```python
from build123d import *

# Parameters (mm, degrees)
MAIN_BODY_DEPTH          = 30.5
SKETCH2_R                = 4.23
LONG_SHAFT_COLLAR_DEPTH  = 2
SKETCH3_R                = 1
LONG_SHAFT_DEPTH         = 10.3
SKETCH5_W                = 8.3
SKETCH5_H                = 5.6
LEAD_BUMP_DEPTH          = 1.15
SKETCH6_R                = 3.075
SHORT_SHAFT_COLLAR_DEPTH = 1.5
SHORT_START              = 5.5
SKETCH7_R                = 1
SHORT_SHAFT_DEPTH        = 5.5


with BuildPart() as part:
    # Sketch1 → Main Body (new body)
    with BuildSketch(Plane.XY):
        with BuildLine():
            Line((-7.867656894, -9.16), (7.867656894, -9.16))
            ThreePointArc((7.867656894, -9.16), (12.075, 0), (7.867656894, 9.16))
            Line((7.867656894, 9.16), (-7.867656894, 9.16))
            ThreePointArc((-7.867656894, 9.16), (-12.075, 0), (-7.867656894, -9.16))
        make_face()
    extrude(amount=MAIN_BODY_DEPTH)

    # Sketch2 → Long Shaft Collar (add)
    with BuildSketch(Plane(origin=(0, 0, 0), x_dir=(-1, 0, 0), z_dir=(0, 0, -1))):
        Circle(SKETCH2_R)
    extrude(amount=LONG_SHAFT_COLLAR_DEPTH)

    # Sketch3 → Long Shaft (add)
    with BuildSketch(Plane(origin=(0, 0, -2), x_dir=(-1, 0, 0), z_dir=(0, 0, -1))):
        with Locations(Location((0, 0, 0), (0, 0, 180))):
            Circle(SKETCH3_R)
    extrude(amount=LONG_SHAFT_DEPTH)

    # Sketch5 → Lead Bump (add)
    with BuildSketch(Plane(origin=(0, 9.16, 0), x_dir=(1, 0, 0), z_dir=(0, 1, 0))):
        with Locations((0, -2.8)):
            Rectangle(SKETCH5_W, SKETCH5_H)
    extrude(amount=LEAD_BUMP_DEPTH)

    # Sketch6 → Short Shaft Collar (add)
    with BuildSketch(Plane.XY.offset(30.5)):
        Circle(SKETCH6_R)
    extrude(amount=SHORT_SHAFT_COLLAR_DEPTH)

    # Sketch7 → Short shaft (add)
    with BuildSketch(Plane.XY.offset(32).offset(SHORT_START)):
        Circle(SKETCH7_R)
    extrude(amount=-SHORT_SHAFT_DEPTH)


solid = part.part
```
Geometry check sheet. Reference: the model listing, model coordinates, mm. A direction names the side the tool comes from. Give positions to 0.01 mm unless a question says otherwise; leave off trailing zeros. Loops run counter-clockwise (first coordinate to the right, second up) from the corner with the lowest first, then second, coordinate; pieces in that order, holes last. Notation, with made-up numbers: M 45,57 L 81,57 A18 ccw 81,61 Z; hole C -37.5,64.5 d2. An arc over 180 degrees is marked long. Write item = value, one per line. Start each with the question number.
1. Thickness scan on probe 1 along Z at (x, y) = (-8.5, 3.75); probe 2 along Y at (x, z) = (4.5, 18); probe 3 along X at (y, z) = (-1, 4). Record the ranges inside material, lowest first.
2. Section check B-B, the plane y = 0. Enter the section's corners in (x, z) (3 decimals).
3. Section check C-C, the plane z = 26.5. Enter the section's corners in (x, y) (3 decimals).
4. Section check D-D, the plane z = -8.5. Enter the section's corners in (x, y).
5. Go/stop test with flat-tipped pins: P1, Ø0.6, axis at x = 1.5, y = 9.5, coming from the +Z side; P2, Ø1.3, axis at y = 9.5, z = 3.5, coming from the -X side; P3, Ø8, axis at x = 6.5, y = 7, coming from the +Z side; P4, Ø1, axis at y = 6, z = -2, coming from the -X side. Record where each tip stops, or that it passes through.
6. Tool access check on faces 1 (the face through (-4.15, 10, 3)), 2 (the face through (3, 2, 30.5)), 3 (the face through (3.36, -2.57, -0.99)). Record the directions out of +Z, -Z, +X, -X, +Y, -Y that give a thin tool (end or side, any length) a straight path to the whole face; none if there is none.
7. Section check A-A, the plane x = 0. Enter the section's corners in (y, z) (3 decimals).
Values follow:
q1.probe_1 = 0 to 30.5
q1.probe_2 = -9.16 to 9.16
q1.probe_3 = -12.03 to 12.03
q2.outline = M -12.075,0 L -4.23,0 L -4.23,-2 L -1,-2 L -1,-12.3 L 1,-12.3 L 1,-2 L 4.23,-2 L 4.23,0 L 12.075,0 L 12.075,30.5 L 3.075,30.5 L 3.075,32 L 1,32 L 1,37.5 L -1,37.5 L -1,32 L -3.075,32 L -3.075,30.5 L -12.075,30.5 Z
q3.outline = M -7.868,-9.16 L 7.868,-9.16 A12.075 ccw 7.868,9.16 L -7.868,9.16 A12.075 ccw Z
q4.outline = C 0,0 d2
q5.P1 = 5.6
q5.P2 = -8.21
q5.P3 = 30.5
q5.P4 = through
q6.face_1 = +Z, -Z, -X, +Y
q6.face_2 = +Z
q6.face_3 = -Z
q7.outline = M -9.16,0 L -4.23,0 L -4.23,-2 L -1,-2 L -1,-12.3 L 1,-12.3 L 1,-2 L 4.23,-2 L 4.23,0 L 10.31,0 L 10.31,5.6 L 9.16,5.6 L 9.16,30.5 L 3.075,30.5 L 3.075,32 L 1,32 L 1,37.5 L -1,37.5 L -1,32 L -3.075,32 L -3.075,30.5 L -9.16,30.5 Z
